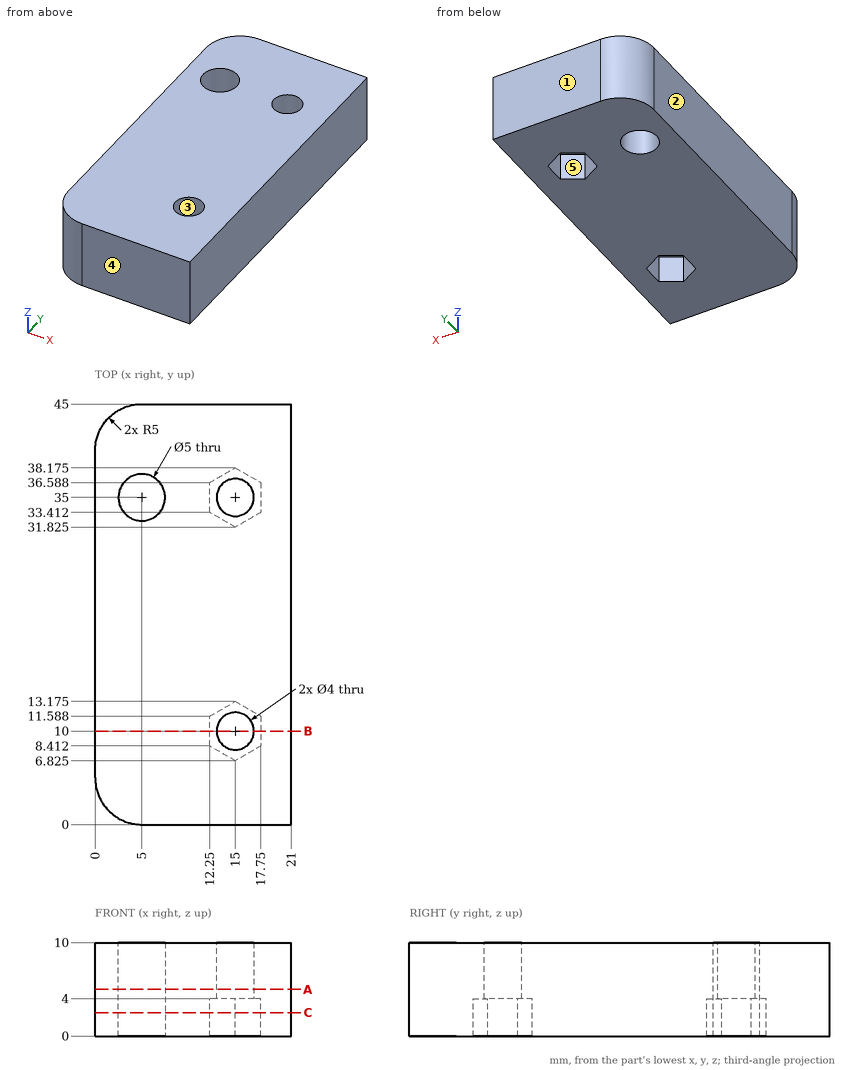
The figure shows three views and two pictorial views of one solid part (mm, origin at its lowest corner). Answer the questions. A direction names the side the tool comes from. Coordinates: 2 decimals unless noted, no trailing zeros. Loops run counter-clockwise (first coordinate to the right, second up) from the corner with the lowest first, then second, coordinate; pieces in that order, holes last.
1) Find the intervals of material crossed by L1, parallel to Y at x = 15, z = 7.05; L2, parallel to Y at x = 13.5, z = 3.75; L3, parallel to Y at x = 5, z = 8.25, in increasing order.
2) Find section C-C on z = 2.5. Give the number of separate pieces and of enclosed holes in the cut face, then the cut area to 3 significant figures.
3) Find section A-A on z = 5. Write down the section's boundary in (x, y).
4) A flat-ended cylindrical pin translates along its axis: pin 1 Ø3 at (x, y) = (15, 35) entering from +Z. Find the tip coordinate at first contact, or state that the pin passes through.
5) Find section B-B on y = 10. Write down the section's boundary in (x, z).
6) Determine the mould class of the marked faces 1, 2 and 3 for opening direction Y: pulls with the +Y half, pulls with the -Y half, needs draft (parallel to the pull), parting line crosses it, or undercut.
7) A tool of negligible diameter and unlimited length cuts with its end or side. For the marked faces 4 and 5, from which of +Z, -Z, +X, -X, +Y, -Y can it reach the whole face along a straight path? Write none if from no direction.
Values:
1. L1: y = 0 to 8, 12 to 33, 37 to 45
1. L2: y = 0 to 7.69, 12.31 to 32.69, 37.31 to 45
1. L3: y = 0 to 32.5, 37.5 to 45
2. separate pieces: 1
2. enclosed holes: 3
2. area: 862 mm2
3. outline: (0, 5) arc R5 ccw to (5, 0) - (21, 0) - (21, 45) - (5, 45) arc R5 ccw to (0, 40) - close; hole circle Ø5 at (5, 35); hole circle Ø4 at (15, 10); hole circle Ø4 at (15, 35)
4. pin 1: passes through
5. outline: (0, 0) - (12.25, 0) - (12.25, 4) - (13, 4) - (13, 10) - (0, 10) - close; (17, 4) - (17.75, 4) - (17.75, 0) - (21, 0) - (21, 10) - (17, 10) - close
6. face 1: pulls with the +Y half
6. face 2: needs draft
6. face 3: undercut
7. face 4: +Z, -Z, +X, -X, -Y
7. face 5: -Z
